The listing builds one solid part. Answer for the finished solid, in the listing's coordinates (mm). Face numbers are marked on the shaded views. A direction names the side the tool comes from. Coordinates: 2 decimals unless noted, no trailing zeros. Loops run counter-clockwise (first coordinate to the right, second up) from the corner with the lowest first, then second, coordinate; pieces in that order, holes last. Notation, with made-up numbers: (8.25, 6) - (65.25, 6) arc R22 cw to (65.25, 39) - close; hole circle Ø5 at (68, 32). An arc over 180 degrees is marked (long way). Return JSON: item names as keys, results as strings. Group by question number.
1. Which of the six approach directions +Z, -Z, +X, -X, +Y, -Y give full straight-line access (tool end or side, diameter ignored) to the marked faces 5 and 6?
2. Section B-B (z = 7) is taken. Write down the section's boundary in (x, y), and give its area (3 significant figures).
3. Section A-A (y = 15) is taken. Write down the section's boundary in (x, z).
4. Find the intervals of material crossed by line 1 along Y through (x, z) = (5, 1.6); line 2 along Z through (x, y) = (5, 0.45); line 3 along Y through (x, z) = (2.25, 8), in increasing order.
5. Each of these flat-tipped pins is pushed along its axis until it touches: P1, Ø2.5, axis at x = 5, y = 15, coming from the +Z side; P2, Ø2, axis at x = 6.5, y = 7, coming from the +Z side. Where does it stop, or does it pass through?
6. Section D-D (x = 0.75) is taken. Write down the section's boundary in (y, z), and give its area (3 significant figures).
7. The mould has two halves that part along X. Classify the marked faces 1, 2, 3 and 4: pulls with the +X half, pulls with the -X half, needs draft (parallel to the pull), parting line crosses it, or undercut.
8. Section C-C (z = 2.25) is taken. Write down the section's boundary in (x, y), and give its area (3 significant figures).
Autodesk Inventor part; units mm, degrees
ref_plane "YZ Plane" through (0, 0, 0) normal (1, 0, 0) x (0, 1, 0)
ref_plane "XZ Plane" through (0, 0, 0) normal (0, 1, 0) x (-1, 0, 0)
ref_plane "XY Plane" through (0, 0, 0) normal (0, 0, 1) x (1, 0, 0)
sketch "Sketch1" plane through (0, 0, 0) normal (0, 0, 1) x (1, 0, 0)
  line L0 (0, 0) -> (10, 0)
  line L1 (10, 0) -> (10, 20)
  line L2 (10, 20) -> (0, 20)
  line L3 (0, 20) -> (0, 0)
  circle A0 centre (5, 15) radius 1.5
  dimension "d0" = 10
  dimension "d1" = 20
  dimension "d8" = 3
  dimension "d19" = 5
  dimension "d20" = 15
extrude "Extrusion1" add sketch "Sketch1" along normal blind 3
sketch "Sketch4" plane through (0, 0, 3) normal (0, 0, 1) x (1, 0, 0)
  line L0 (10, 0) -> (10, 20)
  line L1 (0, 0) -> (10, 0)
  line L2 (10, 0) -> (10, 2)
  line L3 (10, 2) -> (0, 2)
  line L4 (0, 2) -> (0, 0)
  dimension "d9" = 2
extrude "Extrusion2" add sketch "Sketch4" along normal blind 7
sketch "Sketch5" plane through (0, 0, 0) normal (0, -1, 0) x (1, 0, 0)
  circle A0 centre (5, 7) radius 1
  line L0 (10, 0) -> (10, 10)
  line L1 (0, 0) -> (0, 10)
  line L2 (0, 0) -> (10, 0)
  line L3 (0, 10) -> (10, 10)
  dimension "d12" = 10
  dimension "d13" = 10
  dimension "d14" = 7
  dimension "d15" = 5
  dimension "d16" = 2
extrude "Extrusion3" cut sketch "Sketch5" against normal through all contours A0
equation "\"d19\" = 0.5 * d0"
equation "\"d20\" = 0.75 * d1"
equation "\"d15\" = 0.5 * d12"
properties part number "supportPoulie" material "Stainless Steel"
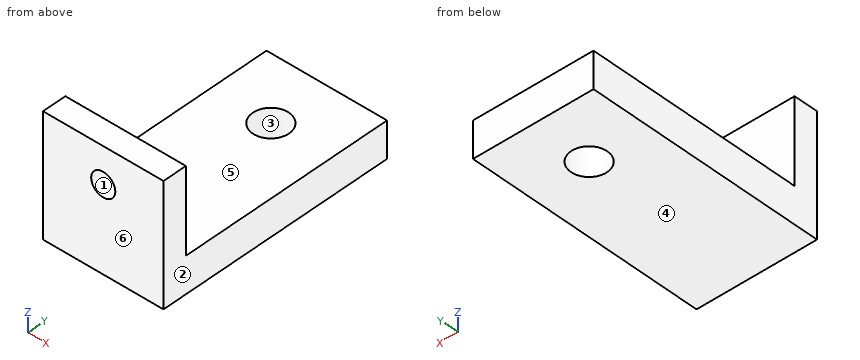
The answers:
{
 "1": {"face 5": "+Z, +X, -X, +Y", "face 6": "+Z, -Z, +X, -X, -Y"},
 "2": {"outline": "(0, 0) - (4, 0) - (4, 2) - (0, 2) - close; (6, 0) - (10, 0) - (10, 2) - (6, 2) - close", "area": "16.0 mm2"},
 "3": {"outline": "(0, 0) - (3.5, 0) - (3.5, 3) - (0, 3) - close; (6.5, 0) - (10, 0) - (10, 3) - (6.5, 3) - close"},
 "4": {"line 1": "y = 0 to 13.5, 16.5 to 20", "line 2": "z = 0 to 6, 8 to 10", "line 3": "y = 0 to 2"},
 "5": {"P1": "passes through", "P2": "stops at z = 3"},
 "6": {"outline": "(0, 0) - (20, 0) - (20, 3) - (2, 3) - (2, 10) - (0, 10) - close", "area": "74.0 mm2"},
 "7": {"face 1": "undercut", "face 2": "pulls with the +X half", "face 3": "undercut", "face 4": "needs draft"},
 "8": {"outline": "(0, 0) - (10, 0) - (10, 20) - (0, 20) - close; hole circle Ø3 at (5, 15)", "area": "193 mm2"}
}
